Here's how the part is built. I have some questions about the finished solid (model axes, mm). A direction names the side the tool comes from. Coordinates: 2 decimals unless noted, no trailing zeros. Write each loop counter-clockwise with the first axis right and the second up, starting at its lowest first coordinate (ties: lowest second). Pieces come first, ordered by that corner, then holes. Notation, with made-up numbers: (32, 71) -> (80, 71) arc R34 cw to (80, 108) -> close; hole circle Ø4 at (46.25, 64.5). An arc over 180 degrees is marked (long way). Put each result on its own line as item: value.
```python
from build123d import *

# Parameters (mm, degrees)
BOX_W                 = 12
BOX_H                 = 8
BOX_DEPTH             = 23
BOX_ROLL_ANGLE        = 20
TORUS_R               = 3
TORUS_ANGLE           = 180
TORUS_ROLL_ANGLE      = -90
TORUS_PLACEMENT_ANGLE = 180
CYLINDER_R            = 3
CYLINDER_DEPTH        = 30


with BuildPart() as pared:
    # Box → Box (new body)
    with BuildSketch(Plane.XY):
        with Locations((6, 4)):
            Rectangle(BOX_W, BOX_H)
    extrude(amount=BOX_DEPTH)


with BuildPart() as pared_1:
    # Box roll: moved
    add(pared.part.rotate(Axis((0, 0, 0), (1, 0, 0)), BOX_ROLL_ANGLE))


with BuildPart() as pared_2:
    # Box placement: moved
    add(pared_1.part.moved(Location((-6, 4, 10))))


with BuildPart() as torus:
    # Torus → Torus (revolve)
    with BuildSketch(Plane.XZ):
        with Locations((10, 0)):
            Circle(TORUS_R)
    revolve(axis=Axis((0, 0, 0), (0, 0, 1)), revolution_arc=TORUS_ANGLE)


with BuildPart() as torus_1:
    # Torus roll: moved
    add(torus.part.rotate(Axis((0, 0, 0), (1, 0, 0)), TORUS_ROLL_ANGLE))


with BuildPart() as torus_2:
    # Torus placement: moved
    add(torus_1.part.moved(Location((10, 0, 0))).rotate(Axis((10, 0, 0), (0, 0, 1)), TORUS_PLACEMENT_ANGLE))


with BuildPart() as cut:
    # Cylinder → Cylinder (new body)
    with BuildSketch(Plane.XY):
        Circle(CYLINDER_R)
    extrude(amount=CYLINDER_DEPTH)

    # Fusion: union Torus
    add(torus_2.part)

    # Cut: cut pared
    add(pared_2.part, mode=Mode.SUBTRACT)


solid = cut.part
```
Item 1: Imagine slicing it at B-B on z = 4.5. Write out the boundary of the cut face in (x, y).
Output:
outline: circle Ø6 at (0, 0)
Item 2: Imagine slicing it at C-C on y = -2.5. Write out the boundary of the cut face in (x, z).
Output:
outline: (-1.66, 0) arc R11.66 ccw to (21.66, 0) -> (18.34, 0) arc R8.34 cw to (1.66, 0) -> (1.66, 27.86) -> (-1.66, 27.86) -> close
Item 3: Which directions (+Z, -Z, +X, -X, +Y, -Y) give clear straight access to the entire face, cutting with the end or side of a thin tool? Please do faces 1 (the flat face through (-0.042, 0.042, 20.875)), 2 (the cylindrical face through (-0.65, -2.93, 11.24)), 3 (the flat face through (20, 0, 0)).
Output:
face 1: +Z, +X, -X, +Y
face 2: +Z
face 3: +Z, +X, +Y, -Y
Item 4: Please list where these lines run through material, in increasing order: line 1 along X through (y, z) = (0, 18); line 2 along X through (y, z) = (1.25, -5.5); line 3 along Z through (x, y) = (18.75, 2). Write a range as from..to.
Output:
line 1: x = -3..3
line 2: x = -1.48..5.24, 14.76..21.48
line 3: z = -8.55..0
Item 5: For P1, Ø12, axis at x = 6, z = 2.5, coming from the +Y side, with a flat end and sliding along its axis, tell me the tip position at first contact or that it passes through.
Output:
P1: stops at y = 3
Item 6: Imagine slicing it at D-D on z = 26. Write out the boundary of the cut face in (x, y).
Output:
outline: (-2.38, -1.82) arc R3 ccw to (2.38, -1.82) -> close
Item 7: Imagine slicing it at A-A on y = 0.75. Write out the boundary of the cut face in (x, z).
Output:
outline: (-2.9, 0) arc R12.9 ccw to (22.9, 0) -> (17.1, 0) arc R7.1 cw to (2.9, 0) -> (2.9, 18.93) -> (-2.9, 18.93) -> close
